Input: part model. Units: mm. Frame: model coordinates. A direction names the side the tool comes from. Coordinates: 2 decimals unless noted, no trailing zeros. Write each loop counter-clockwise with the first axis right and the second up, starting at its lowest first coordinate (ties: lowest second). Pieces come first, ordered by that corner, then holes. Notation, with made-up numbers: (49, 79) - (86, 79) arc R13 cw to (86, 87) - close; hole circle Ø8 at (72.25, -39.5). An arc over 180 degrees is marked (long way). One line per question, with ' | ' between items. Start each with the question number.
1) Draft query along Z for faces 4 (the cylindrical face through (65.14, -4.88, 1.08)), 5 (the cylindrical face through (67.619, 1.915, 23.381)), 6 (the cylindrical face through (57.605, -34.995, 0.565)). Return one class per face: released by +Z, released by -Z, zero draft, split by the parting line, or undercut.
2) Reachability of faces 1 (the cylindrical face through (17.675, 11.923, 3.755)), 2 (the flat face through (63, 0, -15)), 3 (the flat face through (5, 11, -4)) from +Z, -Z, +X, -X, +Y, -Y: full face, straight path, thin tool, end or side. Return the list, or none.
3) Section query A-A on x = 11.5. Return loops of the section in (y, z).
4) Line query: line 1 (X direction, y = 0, z = 20.5); line 2 (X direction, y = -26.5, z = -8.5); line 3 (Z direction, x = 21, y = 0). Output: solid intervals per line, ascending.
5) First-contact query: P1, Ø7.5, axis at y = 0.5, z = -2, coming from the +X side; P2, Ø8, axis at y = 0, z = 0, coming from the +X side; P3, Ø5, axis at x = 22, y = 13, coming from the +Z side; P4, Ø1.5, axis at y = -8, z = -23.5, coming from the -X side. Flat tips, straight axial feed; report the tip coordinate or a pass-through.
Autodesk Inventor part; units mm, degrees
ref_plane "Plano de trabajo3" through (0, 0, 15) normal (0, 0, 1) x (1, 0, 0)
ref_plane "Plano de trabajo6" through (62.8397, -35, 0) normal (0, 1, 0) x (-1, 0, 0)
ref_plane "YZ Plane" through (0, 0, 0) normal (1, 0, 0) x (0, 1, 0)
sketch "Boceto1" plane through (0, 0, 0) normal (0, 0, 1) x (1, 0, 0)
  line L0 (40, 35) -> (44, 35)
  line L1 (75, 35) -> (75, 0)
  line L2 (40, 12.5) -> (40, 15) construction
  line L3 (0, 0) -> (75, 0)
  line L4 (40, 15) -> (30, 15)
  line L5 (30, 15) -> (30, 12.5)
  line L6 (30, 12.5) -> (40, 12.5) construction
  line L7 (40, 15) -> (40, 35)
  line L8 (3.5, 12.5) -> (3.5, 11.5)
  line L9 (3.5, 11.5) -> (5, 11.5)
  line L10 (5, 11.5) -> (5, 12.5)
  line L11 (5, 12.5) -> (30, 12.5)
  line L12 (3.5, 12.5) -> (5, 12.5) construction
  line L13 (0, 12.5) -> (0, 0)
  line L14 (0, 12.5) -> (3.5, 12.5)
  line L15 (65, 35) -> (65, 0) construction
  line L16 (44, 35) -> (45.3397, 30)
  line L17 (45.3397, 30) -> (49.3397, 30)
  line L18 (49.3397, 30) -> (50.6795, 35)
  line L19 (47.3397, 30) -> (47.3397, 35) construction
  line L20 (47.3397, 35) -> (50.6795, 35) construction
  line L21 (44, 35) -> (47.3397, 35) construction
  line L22 (50.6795, 35) -> (75, 35)
  dimension "d59" = 75
  dimension "d61" = 35
  dimension "d82" = 35
  dimension "d111" = 10
  dimension "d112" = 15
  dimension "d113" = 1.5
  dimension "d114" = 1
  dimension "d115" = 25
  dimension "d130" = 12.5
  dimension "d133" = 10
  dimension "d134" = 2
  dimension "d135" = 105
  dimension "d136" = 105
  dimension "d137" = 5
  dimension "d138" = 4
revolve "Revolución1" add sketch "Boceto1" angle 360 about axis through (0, 0, 0) along (1, 0, 0)
ref_plane "Plano de trabajo3" through (0, 0, 15) normal (0, 0, 1) x (1, 0, 0)
sketch "Boceto3" plane through (0, 0, 15) normal (0, 0, 1) x (1, 0, 0)
  circle A0 centre (63, 0) radius 5
  line L0 (75, -35) -> (75, 35)
  point P0 (0, 0)
  dimension "d14" = 5
  dimension "d132" = 12
extrude "Extrusión1" cut sketch "Boceto3" along normal blind 80
mirror "Simetría1" about plane through (0, 0, 0) normal (0, 0, 1) of "Extrusión1"
sketch "Boceto10" plane through (75, 0, 0) normal (1, 0, 0) x (0, 0, -1)
  circle A0 centre (0, 0) radius 45.5
  circle A1 centre (0, 0) radius 12.5 construction
  circle A2 centre (0, 0) radius 5
  dimension "d116" = 91
  dimension "d117" = 10
extrude "Extrusión11" cut sketch "Boceto10" against normal blind 20 contours A2
thread "Rosca5"
thread "Rosca6"
thread "Rosca7"
ref_plane "Plano de trabajo6" through (62.8397, -35, 0) normal (0, 1, 0) x (-1, 0, 0)
sketch "Boceto15" plane through (62.8397, -35, 0) normal (0, 1, 0) x (-1, 0, 0)
  circle A0 centre (-0.1603, 0) radius 5
  line L0 (-12.1603, 35) -> (-12.1603, -35)
  point P0 (62.8397, 0)
  dimension "d139" = 10
  dimension "d140" = 12
sketch "Boceto16" plane through (0, 0, 0) normal (0, 0, 1) x (1, 0, 0)
  line L0 (50.6795, -35) -> (75, -35)
  line L1 (62.8397, -35) -> (29.2758, 5)
  line L2 (62.8397, -35) -> (62.8397, 5) construction
  point P0 (0, 0)
  dimension "d141" = 40
  dimension "d151" = 5
sweep "Barrido1" cut profiles "Boceto15" path "Boceto16" path curves L1
sketch "Boceto17" plane through (0, 0, 0) normal (-1, 0, 0) x (0, 0, 1)
  circle A0 centre (0, 0) radius 5
  circle A1 centre (0, 0) radius 5
  point P0 (0, 0)
  dimension "d144" = 10
extrude "Extrusión13" cut sketch "Boceto17" against normal up to surface
sketch "Sketch18" plane through (75, 0, 0) normal (1, 0, 0) x (0, 0, -1)
  circle A0 centre (0, 0) radius 35
  line L0 (-32, -14.1774) -> (-32, 14.1774)
  line L1 (32, -14.1774) -> (32, 14.1774)
  point P0 (0, 0)
  dimension "d152" = 32
  dimension "d153" = 32
extrude "Extrusion14" cut sketch "Sketch18" against normal blind 25 contours A0 L1 | L0 A0
properties part number "soporte planetario" material "Acetal Resin, Black"
Answer key:
1) face 4: undercut | face 5: zero draft | face 6: split by the parting line
2) face 1: -X | face 2: -Z | face 3: none
3) outline: circle Ø25 at (0, 0); hole circle Ø10 at (0, 0)
4) line 1: 40 to 58, 68 to 75 | line 2: 40 to 75 | line 3: -12.5 to -5, 5 to 12.5
5) P1: x = 75 | P2: x = 55 | P3: z = 6.78 | P4: x = 40
